```python
from build123d import *

# Parameters (mm, degrees)
PAD044_DEPTH         = 79.56
PAD045_DEPTH         = 2
SKETCH132_R          = 5
SKETCH132_W          = 20
SKETCH132_H          = 13
PAD046_DEPTH         = 2
FILLET011_R          = 2
SKETCH133_W          = 9.65
SKETCH133_H          = 4.8
PAD047_DEPTH         = 46
SKETCH134_R          = 1.75
POCKET055_DEPTH      = 46.001
SKETCH135_R          = 1.75
POCKET056_DEPTH      = 5.001
SKETCH136_R          = 3
POCKET057_DEPTH      = 2.951
SKETCH137_R          = 3.2
SKETCH137_R_2        = 1.75
PAD048_DEPTH         = 2.2
SKETCH138_W          = 5.65
SKETCH138_H          = 2.75
POCKET058_DEPTH      = 35.151
POCKET058_DEPTH_BACK = 35.151
PAD049_DEPTH         = 4


with BuildPart() as part:
    # Sketch130 → Pad044 (new body)
    with BuildSketch(Plane.YZ.offset(38.302)):
        with BuildLine():
            ThreePointArc((-33.15, 1), (-32.857107, 0.292893), (-32.15, 0))
            Line((32.15, 0), (-32.15, 0))
            ThreePointArc((32.15, 0), (32.857107, 0.292893), (33.15, 1))
            Line((33.15, 46), (33.15, 1))
            Line((35.15, 46), (33.15, 46))
            Line((35.15, -2), (35.15, 46))
            Line((32.15, -5), (35.15, -2))
            Line((-32.15, -5), (32.15, -5))
            Line((-35.15, -2), (-32.15, -5))
            Line((-35.15, 46), (-35.15, -2))
            Line((-33.15, 46), (-35.15, 46))
            Line((-33.15, 1), (-33.15, 46))
        make_face()
    extrude(amount=-PAD044_DEPTH)

    # Sketch131 → Pad045 (join)
    with BuildSketch(Plane.YZ.offset(38.302)):
        with BuildLine():
            ThreePointArc((-34.05, 1), (-33.493503, -0.343503), (-32.15, -0.9))
            Line((-32.15, -0.9), (32.15, -0.9))
            ThreePointArc((32.15, -0.9), (33.493503, -0.343503), (34.05, 1))
            Line((34.05, 1), (34.05, 46))
            Line((34.05, 46), (33.15, 46))
            Line((33.15, 46), (33.15, 1))
            ThreePointArc((32.15, 0), (32.857107, 0.292893), (33.15, 1))
            Line((32.15, 0), (-32.15, 0))
            ThreePointArc((-33.15, 1), (-32.857107, 0.292893), (-32.15, 0))
            Line((-33.15, 46), (-33.15, 1))
            Line((-34.05, 46), (-33.15, 46))
            Line((-34.05, 46), (-34.05, 1))
        make_face()
    extrude(amount=PAD045_DEPTH)

    # Sketch132 → Pad046 (join)
    with BuildSketch(Plane.YZ.offset(-41.258)):
        with BuildLine():
            ThreePointArc((-33.15, 1), (-32.857107, 0.292893), (-32.15, 0))
            Line((-32.15, 0), (32.15, 0))
            ThreePointArc((32.15, 0), (32.857107, 0.292893), (33.15, 1))
            Line((33.15, 1), (33.15, 46))
            Line((33.15, 46), (-33.15, 46))
            Line((-33.15, 46), (-33.15, 1))
        make_face()
        with Locations((0, 12)):
            Circle(SKETCH132_R, mode=Mode.SUBTRACT)
        with Locations((0, 32.5)):
            Rectangle(SKETCH132_W, SKETCH132_H, mode=Mode.SUBTRACT)
    extrude(amount=PAD046_DEPTH)

    # Fillet011
    fillet011_edges = [part.edges().sort_by_distance(p)[0] for p in [
        (-41.258, 35.15, 22),
        (-41.258, 33.65, -3.5),
        (-41.258, 0, -5),
        (-41.258, -33.65, -3.5),
        (-41.258, -35.15, 22),
    ]]
    fillet(fillet011_edges, radius=FILLET011_R)

    # Sketch133 → Pad047 (join)
    with BuildSketch(Plane.XY):
        with Locations((-4.083, 30.75)):
            Rectangle(SKETCH133_W, SKETCH133_H)
        with Locations((-4.083, -30.75)):
            Rectangle(SKETCH133_W, SKETCH133_H)
    extrude(amount=PAD047_DEPTH)

    # Sketch134 → Pocket055 (cut, through all)
    with BuildSketch(Plane.XY):
        with Locations((-4.083, 31.75)):
            Circle(SKETCH134_R)
        with Locations((-4.083, -31.75)):
            Circle(SKETCH134_R)
    extrude(amount=POCKET055_DEPTH, mode=Mode.SUBTRACT)

    # Sketch135 → Pocket056 (cut, through all)
    with BuildSketch(Plane.XY):
        with Locations((-20.908, 22.75)):
            Circle(SKETCH135_R)
        with Locations((-3.608, 22.75)):
            Circle(SKETCH135_R)
        with Locations((14.696, 24.888)):
            Circle(SKETCH135_R)
        with Locations((31.952, 15.621)):
            Circle(SKETCH135_R)
        with Locations((31.952, -19.431)):
            Circle(SKETCH135_R)
        with Locations((23.841, -28.448)):
            Circle(SKETCH135_R)
        with Locations((5.551, -28.448)):
            Circle(SKETCH135_R)
        with Locations((-3.608, -22.75)):
            Circle(SKETCH135_R)
        with Locations((-20.908, -22.75)):
            Circle(SKETCH135_R)
    extrude(amount=-POCKET056_DEPTH, mode=Mode.SUBTRACT)

    # Sketch136 → Pocket057 (cut, through all)
    with BuildSketch(Plane.XY.offset(-2.05)):
        with Locations((-20.908, 22.75)):
            Circle(SKETCH136_R)
        with Locations((-3.608, 22.75)):
            Circle(SKETCH136_R)
        with Locations((14.696, 24.888)):
            Circle(SKETCH136_R)
        with Locations((31.952, 15.621)):
            Circle(SKETCH136_R)
        with Locations((31.952, -19.431)):
            Circle(SKETCH136_R)
        with Locations((23.841, -28.448)):
            Circle(SKETCH136_R)
        with Locations((5.551, -28.448)):
            Circle(SKETCH136_R)
        with Locations((-3.608, -22.75)):
            Circle(SKETCH136_R)
        with Locations((-20.908, -22.75)):
            Circle(SKETCH136_R)
    extrude(amount=-POCKET057_DEPTH, mode=Mode.SUBTRACT)

    # Sketch137 → Pad048 (join)
    with BuildSketch(Plane.XY):
        with Locations((-20.908, 22.75)):
            Circle(SKETCH137_R)
        with Locations((-20.908, 22.75)):
            Circle(SKETCH137_R_2, mode=Mode.SUBTRACT)
        with Locations((-3.608, 22.75)):
            Circle(SKETCH137_R)
        with Locations((-3.608, 22.75)):
            Circle(SKETCH137_R_2, mode=Mode.SUBTRACT)
        with Locations((14.696, 24.888)):
            Circle(SKETCH137_R)
        with Locations((14.696, 24.888)):
            Circle(SKETCH137_R_2, mode=Mode.SUBTRACT)
        with Locations((23.841, -28.448)):
            Circle(SKETCH137_R)
        with Locations((23.841, -28.448)):
            Circle(SKETCH137_R_2, mode=Mode.SUBTRACT)
        with Locations((5.551, -28.448)):
            Circle(SKETCH137_R)
        with Locations((5.551, -28.448)):
            Circle(SKETCH137_R_2, mode=Mode.SUBTRACT)
        with Locations((-3.608, -22.75)):
            Circle(SKETCH137_R)
        with Locations((-3.608, -22.75)):
            Circle(SKETCH137_R_2, mode=Mode.SUBTRACT)
        with Locations((-20.908, -22.75)):
            Circle(SKETCH137_R)
        with Locations((-20.908, -22.75)):
            Circle(SKETCH137_R_2, mode=Mode.SUBTRACT)
    extrude(amount=PAD048_DEPTH)

    # Sketch138 → Pocket058 (cut, two sides)
    with BuildSketch(Plane.XZ) as pocket058_sk:
        with Locations((-4.083, 40.625)):
            Rectangle(SKETCH138_W, SKETCH138_H)
    extrude(amount=-POCKET058_DEPTH, mode=Mode.SUBTRACT)
    extrude(pocket058_sk.sketch, amount=POCKET058_DEPTH_BACK, mode=Mode.SUBTRACT)

    # Sketch139 → Pad049 (join)
    with BuildSketch(Plane.YZ.offset(40.302)):
        Polygon((-33.15, 46), (-28.35, 46), (-28.35, 36), (-33.15, 31.2), align=None)
        Polygon((33.15, 46), (28.35, 46), (28.35, 36), (33.15, 31.2), align=None)
    extrude(amount=-PAD049_DEPTH)


solid = part.part
```
Verification items for the finished model (mm, model axes). A direction names the side the tool comes from. Coordinates: 2 decimals unless noted, no trailing zeros. Write each loop counter-clockwise with the first axis right and the second up, starting at its lowest first coordinate (ties: lowest second). Pieces come first, ordered by that corner, then holes. Notation, with made-up numbers: (52.25, -39) - (102.25, -39) arc R18 cw to (102.25, -33) - close; hole circle Ø9 at (-24.5, -13.75). An arc over 180 degrees is marked (long way). One line per question, with ' | ' between items. Start each with the question number.
1. Material ranges on line 1 along X through (y, z) = (-22, -3); line 2 along Y through (x, z) = (25, 10); line 3 along X through (y, z) = (-22, -1), recorded low to high.
2. Gauge pin test, flat ends, axial feed: P1, Ø5.5, axis at x = 5.551, y = -28.448, coming from the +Z side; P2, Ø4, axis at y = 4.5, z = 36.5, coming from the +X side; P3, Ø6, axis at y = 8, z = 29.5, coming from the +X side; P4, Ø5.5, axis at x = -3.608, y = 22.75, coming from the -Z side. Record the tip position at first contact, or that the pin passes through.
3. Section check A-A (z = 12). Enter the section's corners in (x, y).
4. Section check B-B (z = 28). Enter the section's corners in (x, y).
5. Draft check along Y on faces 6 (the flat face through (0.06, -33.67, -3.48)), 7 (the cylindrical face through (-3.1, 33.2, 19.4)), 8 (the cylindrical face through (39.288, 33.479, -0.358)). Enter one of: released by +Y, released by -Y, zero draft, split by the parting line, or undercut.
6. Section check C-C (x = -25.5). Enter the section's corners in (y, z), plus the area to 3 significant figures.
7. Access from +Z, -Z, +X, -X, +Y, -Y to the whole of each face (thin tool, end or side, straight path). Record for faces 1 (the flat face through (-19.5, -24.1, 2.2)), 2 (the flat face through (-2, -32, 39.25)), 3 (the flat face through (-40, 0, 39)), 4 (the flat face through (-8.908, -31, 23)), 5 (the flat face through (38.33, -30.72, 33.63)).
Computed values:
1) line 1: -41.26 to -23.81, -18 to -6.51, -0.7 to 30.4, 33.5 to 38.3 | line 2: -35.15 to -33.15, 33.15 to 35.15 | line 3: -41.26 to -22.49, -19.33 to -5.19, -2.03 to 38.3
2) P1: z = 2.2 | P2: through | P3: x = -39.26 | P4: z = -2.05
3) outline: (-41.26, -33.15) arc R2 ccw to (-39.26, -35.15) - (38.3, -35.15) - (38.3, -34.05) - (40.3, -34.05) - (40.3, -33.15) - (0.74, -33.15) - (0.74, -28.35) - (-8.91, -28.35) - (-8.91, -33.15) - (-39.26, -33.15) - (-39.26, -5) - (-41.26, -5) - close; (-41.26, 5) - (-39.26, 5) - (-39.26, 33.15) - (-8.91, 33.15) - (-8.91, 28.35) - (0.74, 28.35) - (0.74, 33.15) - (40.3, 33.15) - (40.3, 34.05) - (38.3, 34.05) - (38.3, 35.15) - (-39.26, 35.15) arc R2 ccw to (-41.26, 33.15) - close; hole circle Ø3.5 at (-4.08, -31.75); hole circle Ø3.5 at (-4.08, 31.75)
4) outline: (-41.26, -33.15) arc R2 ccw to (-39.26, -35.15) - (38.3, -35.15) - (38.3, -34.05) - (40.3, -34.05) - (40.3, -33.15) - (0.74, -33.15) - (0.74, -28.35) - (-8.91, -28.35) - (-8.91, -33.15) - (-39.26, -33.15) - (-39.26, -10) - (-41.26, -10) - close; (-41.26, 10) - (-39.26, 10) - (-39.26, 33.15) - (-8.91, 33.15) - (-8.91, 28.35) - (0.74, 28.35) - (0.74, 33.15) - (40.3, 33.15) - (40.3, 34.05) - (38.3, 34.05) - (38.3, 35.15) - (-39.26, 35.15) arc R2 ccw to (-41.26, 33.15) - close; hole circle Ø3.5 at (-4.08, -31.75); hole circle Ø3.5 at (-4.08, 31.75)
5) face 6: released by -Y | face 7: undercut | face 8: released by +Y
6) outline: (-35.15, -2) - (-32.15, -5) - (32.15, -5) - (35.15, -2) - (35.15, 46) - (33.15, 46) - (33.15, 1) arc R1 cw to (32.15, 0) - (-32.15, 0) arc R1 cw to (-33.15, 1) - (-33.15, 46) - (-35.15, 46) - close | area: 527 mm²
7) face 1: +Z, +X | face 2: +Y, -Y | face 3: +X, -X | face 4: +Z | face 5: +X
